from build123d import *

# Parameters (mm, degrees)
SKETCH1_W                                       = 200
SKETCH1_H                                       = 55
BOSS_EXTRUDE1_DEPTH                             = 30
SKETCH2_W                                       = 8
SKETCH2_H                                       = 20
BOSS_EXTRUDE2_DEPTH                             = 13
SKETCH7_R                                       = 1.25
CUT_EXTRUDE1_DEPTH                              = 49.984212522
SKETCH11_R                                      = 1.25
CUT_EXTRUDE2_DEPTH                              = 13
SKETCH13_W                                      = 71.503175403
SKETCH13_H                                      = 55
SKETCH13_W_2                                    = 71.456081763
BOSS_EXTRUDE3_DEPTH                             = 13
BOSS_EXTRUDE4_DEPTH                             = 55
CSK_FOR_M6_FLAT_HEAD_MACHINE_SCREW2_D           = 6.6
CSK_FOR_M6_FLAT_HEAD_MACHINE_SCREW2_CSINK_D     = 12.6
CSK_FOR_M6_FLAT_HEAD_MACHINE_SCREW2_CSINK_ANGLE = 90


with BuildPart() as part:
    # Sketch1 → Boss-Extrude1 (new body)
    with BuildSketch(Plane(origin=(0, 0, 0), x_dir=(1, 0, 0), z_dir=(0, 1, 0))):
        Rectangle(SKETCH1_W, SKETCH1_H)
    extrude(amount=BOSS_EXTRUDE1_DEPTH)

    # Sketch2 → Boss-Extrude2 (add)
    with BuildSketch(Plane.XZ):
        with Locations((-24.5, 11.484212522)):
            Rectangle(SKETCH2_W, SKETCH2_H)
        with Locations((24.5, 11.484212522)):
            Rectangle(SKETCH2_W, SKETCH2_H)
    extrude(amount=BOSS_EXTRUDE2_DEPTH)

    # Sketch7 → Cut-Extrude1 (cut, through all)
    with BuildSketch(Plane.XY.offset(21.484212522)):
        with Locations((-24.5, -1.5)):
            Circle(SKETCH7_R)
        with Locations((-24.5, -11.5)):
            Circle(SKETCH7_R)
    extrude(amount=-CUT_EXTRUDE1_DEPTH, mode=Mode.SUBTRACT)

    # Sketch11 → Cut-Extrude2 (cut)
    with BuildSketch(Plane.XY.offset(21.484212522)):
        with Locations((24.5, -1.5)):
            Circle(SKETCH11_R)
        with Locations((24.5, -11.5)):
            Circle(SKETCH11_R)
    extrude(amount=-CUT_EXTRUDE2_DEPTH, mode=Mode.SUBTRACT)

    # Sketch13 → Boss-Extrude3 (add)
    with BuildSketch(Plane.XZ):
        with Locations((-64.248412298, 0)):
            Rectangle(SKETCH13_W, SKETCH13_H)
        with Locations((64.271959119, 0)):
            Rectangle(SKETCH13_W_2, SKETCH13_H)
    extrude(amount=BOSS_EXTRUDE3_DEPTH)

    # Sketch26 → Boss-Extrude4 (add, through all)
    with BuildSketch(Plane.XY.offset(27.5)):
        with BuildLine():
            Line((100, -24.02177079), (100, -13))
            Line((100, -13), (28.543918237, -13))
            ThreePointArc((28.543918237, -13), (64.542951108, -16.753996588), (100, -24.02177079))
        make_face()
        with BuildLine():
            Line((-100, -24.02177079), (-100, -13))
            Line((-100, -13), (-28.543918237, -13))
            ThreePointArc((-28.543918237, -13), (-64.542951108, -16.753996588), (-100, -24.02177079))
        make_face()
    extrude(amount=-BOSS_EXTRUDE4_DEPTH)

    # CSK for M6 Flat Head Machine Screw2 (through all)
    with Locations(Plane(origin=(-64.248412299, 30, -17.95872272), x_dir=(0, 0, 1), z_dir=(0, 1, 0))):
        with Locations((0, 0), (0, 128.520371417), (19.47835626, 0), (19.47835626, 128.520371417)):
            CounterSinkHole(CSK_FOR_M6_FLAT_HEAD_MACHINE_SCREW2_D / 2, CSK_FOR_M6_FLAT_HEAD_MACHINE_SCREW2_CSINK_D / 2, counter_sink_angle=CSK_FOR_M6_FLAT_HEAD_MACHINE_SCREW2_CSINK_ANGLE)


solid = part.part
Verification items for the finished model (mm, model axes). A direction names the side the tool comes from. Coordinates: 2 decimals unless noted, no trailing zeros. Loops run counter-clockwise (first coordinate to the right, second up) from the corner with the lowest first, then second, coordinate; pieces in that order, holes last. Notation, with made-up numbers: (51.25, -12) -> (96.25, -12) arc R23 cw to (96.25, 8) -> close; hole circle Ø3 at (8, 41). An arc over 180 degrees is marked (long way). Answer as a JSON object with one key per item and string values. Group by question number.
Item 1: Sectioned sample at D-D on x = -83. Record the boundary of the cut face in (y, z), plus the area to 3 significant figures.
Item 2: Mould release check, pull along Z, two halves, no side actions. Record for faces 1 (the conical face through (-67.612, 27.146, -17.212)), 2 (the conical face through (67.18, 27.15, -19.81)), 3 (the flat face through (24, -6, 21.484)), 4 (the flat face through (-28.497, -6, -13)): +Z half, -Z half, draft (parallel to the pull), parting line (faces both ways), or undercut.
Item 3: Sectioned sample at B-B on x = 3.5. Record the boundary of the cut face in (y, z), plus the area to 3 significant figures.
Item 4: Tool access check on faces 5 (the flat face through (-28.497, -6, 24)), 6 (the flat face through (24, -6, 1.484)), 7 (the flat face through (20.5, -6, 11)). Record the directions out of +Z, -Z, +X, -X, +Y, -Y that give a thin tool (end or side, any length) a straight path to the whole face; none if there is none.
Item 5: Depth check by flat-ended pin: pin 1 (0.8 mm diameter, centred on x = 24, y = -11.5, fed in from +Z); pin 2 (4 mm diameter, centred on x = -23.5, z = -5, fed in from -Y); pin 3 (3 mm diameter, centred on x = -24.5, y = -11.5, fed in from -Z); pin 4 (2 mm diameter, centred on x = -24.5, y = -1.5, fed in from -Z). Enter the tip coordinate at first touch or a pass-through.
Item 6: Sectioned sample at C-C on z = -16.5. State how many separate pieces and enclosed holes the cut face has, plus the area to 3 significant figures.
Item 7: Scan lines: probe 1 along Y at (x, z) = (24.5, 19); probe 2 along X at (y, z) = (-6, -18); probe 3 along Y at (x, z) = (24, 15). Record each from-to range of solid material in increasing order.
Item 8: Sectioned sample at A-A on z = 16. Record the boundary of the cut face in (x, y), plus the area to 3 significant figures.
Evaluation:
{
 "1": {"outline": "(-20.08, -27.5) -> (30, -27.5) -> (30, 27.5) -> (-20.08, 27.5) -> close", "area": "2,750 mm²"},
 "2": {"face 1": "undercut", "face 2": "undercut", "face 3": "+Z half", "face 4": "draft"},
 "3": {"outline": "(0, -27.5) -> (30, -27.5) -> (30, 27.5) -> (0, 27.5) -> close", "area": "1,650 mm²"},
 "4": {"face 5": "+Z, -Y", "face 6": "-Z, -Y", "face 7": "+Z, -Z, -Y"},
 "5": {"pin 1": "stops at z = 8.48", "pin 2": "stops at y = 0", "pin 3": "stops at z = 1.48", "pin 4": "passes through"},
 "6": {"separate pieces": "3", "enclosed holes": "0", "area": "7,900 mm²"},
 "7": {"probe 1": "y = -13 to -12.75, -10.25 to -2.75, -0.25 to 30", "probe 2": "x = -100 to -67.55, -60.95 to -28.5, 28.54 to 60.97, 67.57 to 100", "probe 3": "y = -13 to -12.65, -10.35 to -2.65, -0.35 to 30"},
 "8": {"outline": "(-100, -24.02) arc R368.47 cw to (-28.54, -13) -> (-20.5, -13) -> (-20.5, 0) -> (20.5, 0) -> (20.5, -13) -> (28.5, -13) -> (28.5, 0) -> (28.54, 0) -> (28.54, -13) arc R368.47 cw to (100, -24.02) -> (100, 30) -> (-100, 30) -> close; hole circle Ø2.5 at (-24.5, -11.5); hole circle Ø2.5 at (-24.5, -1.5); hole circle Ø2.5 at (24.5, -11.5); hole circle Ø2.5 at (24.5, -1.5)", "area": "8,660 mm²"}
}
